from build123d import *

# Parameters (mm, degrees)
F1_DEPTH = 79.375
F3_D     = 15.875
F3_DEPTH = 50.8
F3_TIP   = 4.7693311635
F5_D     = 6.5278
F5_DEPTH = 20.32
F5_TIP   = 1.9611489744


with BuildPart() as f1:
    # F0 (on Right) → F1 (new body, symmetric)
    with BuildSketch(Plane.YZ):
        Polygon((60.325, 28.0162), (24.8412, 63.5), (-60.325, 63.5), (-60.325, -63.5), (60.325, -63.5), align=None)
    extrude(amount=F1_DEPTH, both=True)

    # F3
    with Locations(Plane.XZ.offset(60.325)):
        with Locations((-38.1, 33.3375), (40.3606, 33.3375), (40.3606, -42.8625)):
            Hole(F3_D / 2, depth=F3_DEPTH)
            with Locations((0, 0, -(F3_DEPTH + F3_TIP / 2))):  # 118° drill point
                Cone(0, F3_D / 2, F3_TIP, mode=Mode.SUBTRACT)

    # F5
    with Locations(Plane.XY.offset(63.5)):
        with Locations((-58.2676, -15.3162), (-58.2676, -47.3202), (-13.2588, -47.3202), (-13.2588, -15.3162)):
            Hole(F5_D / 2, depth=F5_DEPTH)
            with Locations((0, 0, -(F5_DEPTH + F5_TIP / 2))):  # 118° drill point
                Cone(0, F5_D / 2, F5_TIP, mode=Mode.SUBTRACT)


solid = f1.part
The model under review builds one solid part; all positions refer to its coordinate system, in mm. A direction names the side the tool comes from. Coordinates: 2 decimals unless noted, no trailing zeros. Loops run counter-clockwise (first coordinate to the right, second up) from the corner with the lowest first, then second, coordinate; pieces in that order, holes last.
(1) Consider section A-A, the plane z = 47.5. Give the boundary of the cut face in (x, y) (1 decimal).
Determined:
outline: (-79.4, -60.3) - (79.4, -60.3) - (79.4, 40.8) - (-79.4, 40.8) - close; hole circle Ø6.5 at (-58.3, -47.3); hole circle Ø6.5 at (-58.3, -15.3); hole circle Ø6.5 at (-13.3, -47.3); hole circle Ø6.5 at (-13.3, -15.3)
(2) Insertion check: P1, Ø4, axis at x = -58.27, y = -47.32, coming from the +Z side. The pin has a flat end and moves straight along its axis. Give the tip position at first contact, or say it passes through.
Determined:
P1: stops at z = 42.42
(3) Draft analysis for pull direction Y (two halves, no side actions). For faces 1 (the flat face through (1, -17, 63.5)), 2 (the cylindrical face through (-12.834, -44.084, 53.198)), 3 (the flat face through (1.11, 42.83, 45.51)), state which applies: +Y half, -Y half, draft (parallel to the pull), parting line (faces both ways), or undercut.
Determined:
face 1: draft
face 2: undercut
face 3: +Y half
(4) Consider section C-C, the plane x = 17.5. Give the boundary of the cut face in (y, z) (3 decimals).
Determined:
outline: (-60.325, -63.5) - (60.325, -63.5) - (60.325, 28.016) - (24.841, 63.5) - (-60.325, 63.5) - close
(5) Wall thickness on L1, parallel to Z at x = -37.5, y = -30.5; L2, parallel to X at y = -28, z = -45 (3 decimals); L3, parallel to X at y = -19, z = -36.5 (3 decimals): over which ranges is each line inside the solid? List them lowest first.
Determined:
L1: z = -63.5 to 25.42, 41.25 to 63.5
L2: x = -79.375 to 32.716, 48.005 to 79.375
L3: x = -79.375 to 35.615, 45.106 to 79.375
(6) Tool access review of faces 4 (the flat face through (1, 60.325, -18)), 5 (the cylindrical face through (-61.38, -14.34, 53.2)), 6 (the cylindrical face through (36.698, -34.569, -49.904)): name each direction out of +Z, -Z, +X, -X, +Y, -Y from which nothing blocks a thin tool from reaching the whole face with its end or side.
Determined:
face 4: +Z, -Z, +X, -X, +Y
face 5: +Z
face 6: -Y
(7) Consider section B-B, the plane y = -23. Give the boundary of the cut face in (x, z) (1 decimal), plus the area to 3 significant figures.
Determined:
outline: (-79.4, -63.5) - (79.4, -63.5) - (79.4, 63.5) - (-79.4, 63.5) - close; hole circle Ø15.9 at (-38.1, 33.3); hole circle Ø15.9 at (40.4, -42.9); hole circle Ø15.9 at (40.4, 33.3)
area: 19,600 mm2
